Print and shaded views of the part. All mm, measured from the part's lowest x, y and z. A direction names the side the tool comes from. Give positions to 0.01 mm unless a question says otherwise; leave off trailing zeros. Loops run counter-clockwise (first coordinate to the right, second up) from the corner with the lowest first, then second, coordinate; pieces in that order, holes last. Notation, with made-up numbers: (-20, 32) - (5, 32) arc R36 ccw to (5, 69) - close; hole circle Ø11 at (73, 82). An arc over 180 degrees is marked (long way). Return JSON: item names as keys, results as strings.
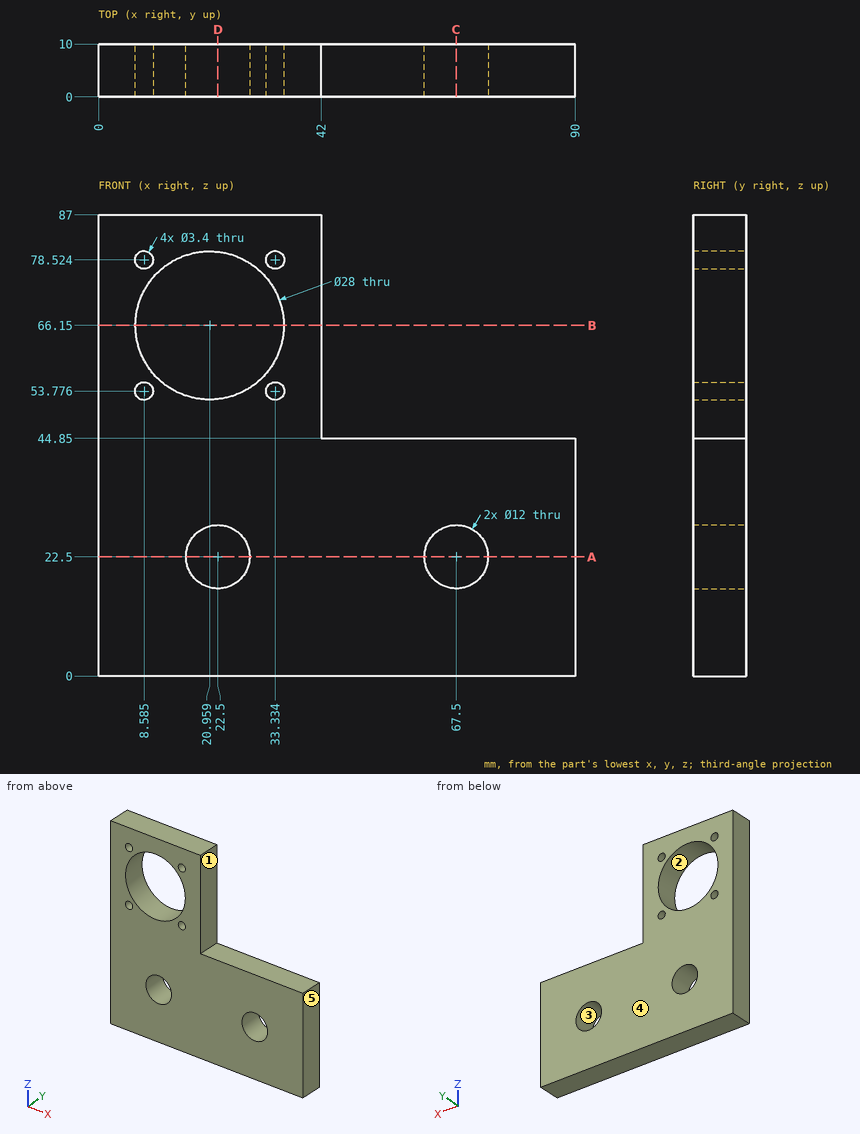
1. Cut at A-A, the plane z = 22.5. Write the cut outline in (x, y).
Values follow:
{"outline": "(0, 0) - (16.5, 0) - (16.5, 10) - (0, 10) - close; (28.5, 0) - (61.5, 0) - (61.5, 10) - (28.5, 10) - close; (73.5, 0) - (90, 0) - (90, 10) - (73.5, 10) - close"}
2. Which spindle directions (+Z, -Z, +X, -X, +Y, -Y) get a long thin tool onto all of the face, cutting with end or side? Do the marked faces 1 and 2. Say none if no direction does.
Values follow:
{"face 1": "+Z, +X, +Y, -Y", "face 2": "+Y, -Y"}
3. Drop flat-ended pins along their axis: P1, Ø2.5, axis at x = 33.33, z = 53.78, coming from the -Y side; P2, Ø5, axis at y = 4, z = 67.5, coming from the +X side. Give the stop position or say it passes through.
Values follow:
{"P1": "passes through", "P2": "stops at x = 42"}
4. Cut at B-B, the plane z = 66.15. Write the cut outline in (x, y), plus the area to 3 significant figures.
Values follow:
{"outline": "(0, 0) - (6.96, 0) - (6.96, 10) - (0, 10) - close; (34.96, 0) - (42, 0) - (42, 10) - (34.96, 10) - close", "area": "140 mm²"}
5. Cut at C-C, the plane x = 67.5. Write the cut outline in (y, z).
Values follow:
{"outline": "(0, 0) - (10, 0) - (10, 16.5) - (0, 16.5) - close; (0, 28.5) - (10, 28.5) - (10, 44.85) - (0, 44.85) - close"}
6. Cut at D-D, the plane x = 22.5. Write the cut outline in (y, z) (1 decimal), plus the area to 3 significant figures.
Values follow:
{"outline": "(0, 0) - (10, 0) - (10, 16.5) - (0, 16.5) - close; (0, 28.5) - (10, 28.5) - (10, 52.2) - (0, 52.2) - close; (0, 80.1) - (10, 80.1) - (10, 87) - (0, 87) - close", "area": "472 mm²"}
7. Pull direction X, two halves, no side cores. Call the marked faces 3, 4 and 5: +X half, -X half, draft (parallel to the pull), parting line (faces both ways), or undercut.
Values follow:
{"face 3": "undercut", "face 4": "draft", "face 5": "+X half"}
8. Drill centre lines: probe 1 along Z at (x, y) = (67.5, 2.75); probe 2 along X at (y, z) = (2.25, 66.15); probe 3 along Z at (x, y) = (22.5, 3) (1 decimal). Where is each one in solid material? Low to high.
Values follow:
{"probe 1": "z = 0 to 16.5, 28.5 to 44.85", "probe 2": "x = 0 to 6.96, 34.96 to 42", "probe 3": "z = 0 to 16.5, 28.5 to 52.2, 80.1 to 87"}
